Part model, mm, in its own coordinate system. Face numbers are marked on the shaded views. Round coordinates to 2 decimals unless told otherwise and drop trailing zeros. Order: outer loops, then holes, each group sorted by start corner. A loop starts at its lowest first (then second) coordinate and runs counter-clockwise, first axis right, second up. Notation, with made-up numbers: (-6.75, -15.75) - (5.25, -15.75) arc R18 cw to (5.25, 8.25) - close; hole circle Ø4 at (86, -38.5). An arc over 180 degrees is marked (long way). Return JSON: item names as keys, results as strings. Group by question number.
Item 1: Saw through at A-A on y = 4. List the corners of the cut face in (x, z).
Item 2: Probe probe 1 along Z at (x, y) = (0, 7.9); probe 2 along X at (y, z) = (0.5, 0); probe 3 along Z at (x, y) = (6.5, 3.75). List the from-to ranges inside material, lowest first.
Item 3: Drop a flat-ended pin along its axis: pin 1 (2.5 mm diameter, centred on x = -8, z = 0, fed in from +Y). Give the stop position or say it passes through.
Item 4: Saw through at C-C on z = 0. List the corners of the cut face in (x, y).
Item 5: Saw through at B-B on x = 0. List the corners of the cut face in (y, z).
Item 6: Saw through at D-D on y = 7.5. List the corners of the cut face in (x, z).
Item 7: Two-plate mould, pull along Z, no slides. Class the marked faces 1, 2 and 3: released by +Z, released by -Z, zero draft, split by the parting line, or undercut.
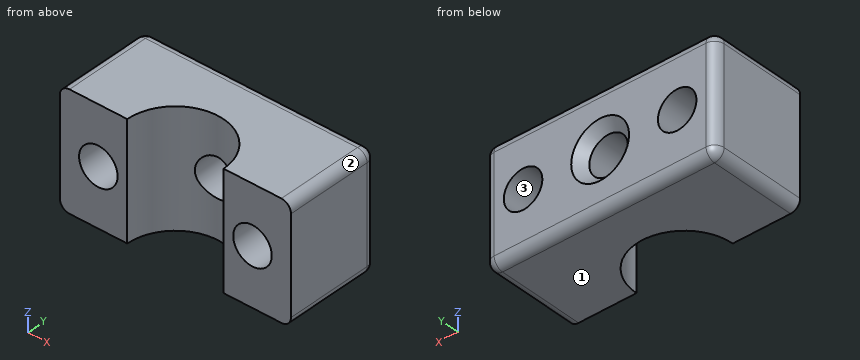
```python
from build123d import *

# Parameters (mm, degrees)
SKETCH1_W           = 24
SKETCH1_H           = 12
SKETCH1_R           = 2
BOSS_EXTRUDE1_DEPTH = 10
CHAMFER1_SIZE       = 1
FILLET1_R           = 1
CUT_EXTRUDE1_DEPTH  = 13


with BuildPart() as part:
    # Sketch1 → Boss-Extrude1 (new body)
    with BuildSketch(Plane(origin=(0, 0, 0), x_dir=(1, 0, 0), z_dir=(0, 1, 0))):
        Rectangle(SKETCH1_W, SKETCH1_H)
        with Locations((8, 0)):
            Circle(SKETCH1_R, mode=Mode.SUBTRACT)
        with Locations((-8, 0)):
            Circle(SKETCH1_R, mode=Mode.SUBTRACT)
        Circle(SKETCH1_R, mode=Mode.SUBTRACT)
    extrude(amount=BOSS_EXTRUDE1_DEPTH)

    # Chamfer1
    chamfer1_edges = [part.edges().sort_by_distance(p)[0] for p in [
        (-2, 10, 0),
    ]]
    chamfer(chamfer1_edges, length=CHAMFER1_SIZE)

    # Fillet1
    fillet1_edges = [part.edges().sort_by_distance(p)[0] for p in [
        (-12, 10, 0),
        (0, 10, 6),
        (12, 10, 0),
        (12, 5, 6),
        (-12, 5, 6),
        (-12, 5, -6),
        (12, 5, -6),
        (0, 10, -6),
    ]]
    fillet(fillet1_edges, radius=FILLET1_R)

    # Sketch2 → Cut-Extrude1 (cut, through all)
    with BuildSketch(Plane(origin=(0, 0, -6), x_dir=(-1, 0, 0), z_dir=(0, 0, -1))):
        with BuildLine():
            Line((-5, 0), (5, 0))
            ThreePointArc((5, 0), (0, 5), (-5, 0))
        make_face()
    extrude(amount=-CUT_EXTRUDE1_DEPTH, mode=Mode.SUBTRACT)


solid = part.part
```
Filled in:
{
 "1": {"outline": "(-12, -5) arc R1 ccw to (-11, -6) - (-3, -6) - (-3, 6) - (-11, 6) arc R1 ccw to (-12, 5) - close; (3, -6) - (11, -6) arc R1 ccw to (12, -5) - (12, 5) arc R1 ccw to (11, 6) - (3, 6) - close; hole circle Ø4 at (-8, 0); hole circle Ø4 at (8, 0)"},
 "2": {"probe 1": "z = -6 to -2, 2 to 6", "probe 2": "x = -12 to -10, -6 to -4.97, 4.97 to 6, 10 to 12", "probe 3": "z = -6 to -1.32, 1.32 to 6"},
 "3": {"pin 1": "passes through"},
 "4": {"outline": "(-12, 0) - (-10, 0) - (-10, 10) - (-11, 10) arc R1 ccw to (-12, 9) - close; (-6, 0) - (-5, 0) arc R5 cw to (-2, 4.58) - (-2, 9) - (-3, 10) - (-6, 10) - close; (2, 4.58) arc R5 cw to (5, 0) - (6, 0) - (6, 10) - (3, 10) - (2, 9) - close; (10, 0) - (12, 0) - (12, 9) arc R1 ccw to (11, 10) - (10, 10) - close"},
 "5": {"outline": "(5, -6) - (9, -6) arc R1 ccw to (10, -5) - (10, -3) - (9, -2) - (5, -2) - close; (5, 2) - (9, 2) - (10, 3) - (10, 5) arc R1 ccw to (9, 6) - (5, 6) - close"},
 "6": {"outline": "(-12, -5) arc R1 ccw to (-11, -6) - (11, -6) arc R1 ccw to (12, -5) - (12, 5) arc R1 ccw to (11, 6) - (-11, 6) arc R1 ccw to (-12, 5) - close; hole circle Ø4 at (-8, 0); hole circle Ø4 at (0, 0); hole circle Ø4 at (8, 0)"},
 "7": {"face 1": "released by -Z", "face 2": "released by +Z", "face 3": "undercut"}
}
